Part model, mm, in its own coordinate system. A direction names the side the tool comes from. Give positions to 0.01 mm unless a question says otherwise; leave off trailing zeros. Order: outer loops, then holes, each group sorted by start corner. A loop starts at its lowest first (then second) coordinate and runs counter-clockwise, first axis right, second up. Notation, with made-up numbers: (55, 43.5) - (95, 43.5) arc R31 cw to (95, 70.5) - close; hole circle Ø11 at (8.5, -6.5). An arc over 180 degrees is marked (long way). One line per item, written item: value.
```python
from build123d import *

# Parameters (mm, degrees)
F0_R     = 17.5
F1_DEPTH = 20
F2_W     = 80
F2_H     = 100
F2_W_2   = 70
F2_H_2   = 90
F3_DEPTH = 1062.5
F6_R     = 2
F7_DEPTH = 5


with BuildPart() as f1:
    # F0 (on Right) → F1 (new body)
    with BuildSketch(Plane.YZ):
        with BuildLine():
            Line((-1206.5, 0), (0, 0))
            Line((0, 0), (0, 100))
            Line((0, 100), (-1123, 100))
            Line((-1123, 100), (-1123, 75))
            ThreePointArc((-1123, 75), (-1143, 55), (-1163, 75))
            Line((-1163, 75), (-1206.5, 75))
            Line((-1206.5, 75), (-1206.5, 0))
        make_face()
        with Locations((-685.8, 50)):
            Circle(F0_R, mode=Mode.SUBTRACT)
    extrude(amount=-F1_DEPTH)

    # F2 (on face) → F3 (join)
    with BuildSketch(Plane(origin=(-20, 0, 0), x_dir=(0, -1, 0), z_dir=(-1, 0, 0))):
        with Locations((40, 50)):
            Rectangle(F2_W, F2_H)
        with Locations((40, 50)):
            Rectangle(F2_W_2, F2_H_2, mode=Mode.SUBTRACT)
    extrude(amount=F3_DEPTH)

    # F5: F1 across plane


with BuildPart() as f1_1:
    add(f1.part)
    add(f1.part.mirror(Plane(origin=(-551.25, -630.0028317099, 49.186434827), x_dir=(0, -1, 0), z_dir=(-1, 0, 0))))

    # F6 (on face) → F7 (cut, through all)
    with BuildSketch(Plane.XZ.offset(80)):
        with Locations((-927.5, 88)):
            Circle(F6_R)
    extrude(amount=-F7_DEPTH, mode=Mode.SUBTRACT)


solid = f1_1.part
```
1) Slice it at D-D on y = -1143. Write the cut outline in (x, z).
Answer:
outline: (-1102.5, 0) - (-1082.5, 0) - (-1082.5, 55) - (-1102.5, 55) - close; (-20, 0) - (0, 0) - (0, 55) - (-20, 55) - close
2) Wall check: line 1 along X through (y, z) = (-771.5, 45); line 2 along Y through (x, z) = (-316, 12.5); line 3 along Z through (x, y) = (-333.5, -69). Give the ranges that are in metal, low to high. Write a range as [from, to].
Answer:
line 1: x = [-1102.5, -1082.5], [-20, 0]
line 2: y = [-80, -75], [-5, 0]
line 3: z = [0, 5], [95, 100]
3) Drop flat-ended pins along their axis: P1, Ø10, axis at x = -1097, y = -1184, coming from the +Z side; P2, Ø16, axis at x = -1093.5, z = 92, coming from the -Y side; P3, Ø10, axis at x = -890.5, z = 17.5, coming from the -Y side. Give the stop position or say it passes through.
Answer:
P1: stops at z = 75
P2: stops at y = -1123
P3: stops at y = -80
4) Slice it at A-A on y = -130. Write the cut outline in (x, z), then the cut area to 3 significant figures.
Answer:
outline: (-1102.5, 0) - (-1082.5, 0) - (-1082.5, 100) - (-1102.5, 100) - close; (-20, 0) - (0, 0) - (0, 100) - (-20, 100) - close
area: 4,000 mm2
5) Slice it at C-C on y = -683. Write the cut outline in (x, z), then the cut area to 3 significant figures.
Answer:
outline: (-1102.5, 0) - (-1082.5, 0) - (-1082.5, 32.73) - (-1102.5, 32.73) - close; (-1102.5, 67.27) - (-1082.5, 67.27) - (-1082.5, 100) - (-1102.5, 100) - close; (-20, 0) - (0, 0) - (0, 32.73) - (-20, 32.73) - close; (-20, 67.27) - (0, 67.27) - (0, 100) - (-20, 100) - close
area: 2,620 mm2
6) Slice it at B-B on x = -452.5. Write the cut outline in (y, z).
Answer:
outline: (-80, 0) - (0, 0) - (0, 100) - (-80, 100) - close; hole (-75, 5) - (-5, 5) - (-5, 95) - (-75, 95) - close
7) Which spindle directions (+Z, -Z, +X, -X, +Y, -Y) get a long thin tool onto all of the face, cutting with end or side? Do faces 1 (the face through (-9.86, -676.392, 64.756)), 2 (the face through (-1082.5, -651, 51)), 3 (the face through (-20, -40, 51)). Say none if no direction does.
Answer:
face 1: +X, -X
face 2: +Z, -Z, -Y
face 3: none
8) Two-plate mould, pull along X, no slides. Class faces 4 (the face through (-544, -80, 49)), 5 (the face through (-385, -64, 0)), 6 (the face through (0, -612, 51)): pulls with the +X half, pulls with the -X half, needs draft (parallel to the pull), parting line crosses it, or undercut.
Answer:
face 4: undercut
face 5: needs draft
face 6: pulls with the +X half
